```python
from build123d import *

# Parameters (mm, degrees)
CHAMFER1_SIZE                 = 1.5
TAP_DRILL_FOR_4_40_TAP1_D     = 2.2606
TAP_DRILL_FOR_4_40_TAP1_DEPTH = 8.89
TAP_DRILL_FOR_4_40_TAP1_TIP   = 0.679152758
TAP_DRILL_FOR_4_40_TAP2_D     = 2.2606
TAP_DRILL_FOR_4_40_TAP2_DEPTH = 8.89
TAP_DRILL_FOR_4_40_TAP2_TIP   = 0.679152758
SKETCH8_R                     = 1.524
CUT_EXTRUDE1_DEPTH            = 8.89
CIRPATTERN1_COUNT             = 6
SKETCH12_W                    = 20.7971
SKETCH12_H                    = 2
CUT_EXTRUDE3_DEPTH            = 2
FILLET1_R                     = 0.5


with BuildPart() as part:
    # Sketch3 → Revolve1 (revolve)
    with BuildSketch(Plane(origin=(0, 0, 0), x_dir=(1, 0, 0), z_dir=(0, 1, 0)), mode=Mode.PRIVATE) as revolve1_sk:
        Polygon((-10.39855, -111.125), (10.39855, -111.125), (10.39855, -107), (5.39855, -107), (5.39855, -100), (1.5875, -100), (1.5875, -101), (-1.5875, -101), (-1.5875, -100), (-5.39855, -100), (-5.39855, -107), (-10.39855, -107), align=None)
    revolve(revolve1_sk.sketch.rotate(Axis((0, 0, 0), (-1, 0, 0)), 180), axis=Axis((0, 0, 0), (-1, 0, 0)))

    # Chamfer1
    chamfer1_edges = [part.edges().sort_by_distance(p)[0] for p in [
        (5.39855, 0, 100),
    ]]
    chamfer(chamfer1_edges, length=CHAMFER1_SIZE)

    # Tap Drill for _4-40 Tap1
    with Locations(Plane(origin=(5.39855, -103.5, 0), x_dir=(0, 0, 1), z_dir=(1, 0, 0))):
        with Locations((0, 0), (89.633629292, -51.75), (-89.633629292, -51.75), (-89.633629292, -155.25), (0, -207), (89.633629292, -155.25)):
            Hole(TAP_DRILL_FOR_4_40_TAP1_D / 2, depth=TAP_DRILL_FOR_4_40_TAP1_DEPTH)
            with Locations((0, 0, -(TAP_DRILL_FOR_4_40_TAP1_DEPTH + TAP_DRILL_FOR_4_40_TAP1_TIP / 2))):  # 118° drill point
                Cone(0, TAP_DRILL_FOR_4_40_TAP1_D / 2, TAP_DRILL_FOR_4_40_TAP1_TIP, mode=Mode.SUBTRACT)

    # Tap Drill for _4-40 Tap2
    with Locations(Plane(origin=(-5.39855, -89.633629292, 51.75), x_dir=(0, 0, -1), z_dir=(-1, 0, 0))):
        with Locations((0, 0), (-51.75, -89.633629292), (0, -179.267258584), (103.5, -179.267258584), (155.25, -89.633629292), (103.5, 0)):
            Hole(TAP_DRILL_FOR_4_40_TAP2_D / 2, depth=TAP_DRILL_FOR_4_40_TAP2_DEPTH)
            with Locations((0, 0, -(TAP_DRILL_FOR_4_40_TAP2_DEPTH + TAP_DRILL_FOR_4_40_TAP2_TIP / 2))):  # 118° drill point
                Cone(0, TAP_DRILL_FOR_4_40_TAP2_D / 2, TAP_DRILL_FOR_4_40_TAP2_TIP, mode=Mode.SUBTRACT)

    # Sketch8 → Cut-Extrude1 (cut)
    with BuildSketch(Plane(origin=(0, 107.338507446, 28.761266387), x_dir=(-1, 0, 0), z_dir=(0, 0.9659258262890681, 0.25881904510252135))):
        with Locations(Location((-2.89855, 0, 0), (0, 0, 90))):
            Circle(SKETCH8_R)
        with Locations(Location((2.89855, 0, 0), (0, 0, 90))):
            Circle(SKETCH8_R)
    cut_extrude1 = extrude(amount=-CUT_EXTRUDE1_DEPTH, mode=Mode.SUBTRACT)

    # CirPattern1: Cut-Extrude1 ×6 about axis
    cirpattern1_axis = Axis((0, 0, 0), (1, 0, 0))
    for i in range(1, CIRPATTERN1_COUNT):
        add(cut_extrude1.rotate(cirpattern1_axis, i * 360 / CIRPATTERN1_COUNT), mode=Mode.SUBTRACT)

    # Sketch12 → Cut-Extrude3 (cut)
    with BuildSketch(Plane(origin=(10.39855, -9.685181913, -110.702135825), x_dir=(-1, 0, 0), z_dir=(0, -0.08715574274765833, -0.9961946980917457))):
        with Locations((10.39855, 1)):
            Rectangle(SKETCH12_W, SKETCH12_H)
        with Locations((10.39855, -1)):
            Rectangle(SKETCH12_W, SKETCH12_H)
    extrude(amount=-CUT_EXTRUDE3_DEPTH, mode=Mode.SUBTRACT)

    # Fillet1
    fillet1_edges = [part.edges().sort_by_distance(p)[0] for p in [
        (0, -11.676002575, -110.509893624),
        (0, -7.691223782, -110.858516595),
        (10.39855, -11.589631199, -109.522664284),
        (10.39855, -7.604852407, -109.871287255),
        (-10.39855, -7.604852407, -109.871287255),
        (-10.39855, -9.510870427, -108.709746429),
        (-10.39855, -11.589631199, -109.522664284),
        (0, -11.503259824, -108.535434944),
        (10.39855, -9.510870427, -108.709746429),
        (0, -7.518481031, -108.884057915),
    ]]
    fillet(fillet1_edges, radius=FILLET1_R)


solid = part.part
```
Model file for the job. Use its own axes, mm. A direction names the side the tool comes from. Coordinates: 2 decimals unless noted, no trailing zeros. Answer as a JSON object with one key per item and string values. Group by question number.
(1) Two-plate mould, pull along Y, no slides. Class faces 5 (the face through (10.399, -91, 58)), 6 (the face through (0.15, 4.84, 111.02)), 7 (the face through (2.73, -30.04, -95.38)), 8 (the face through (-7.93, 65.11, 84.91)): released by +Y, released by -Y, zero draft, split by the parting line, or undercut.
(2) Probe line 1 along Y through (x, z) = (3.4, 0) (3 decimals); line 2 along Y through (x, z) = (-1, -51.75); line 3 along Z through (x, y) = (2.5, 51.75). List the from-to ranges inside material, lowest first.
(3) Tool access for faces 1 (the face through (-10.399, -91, -58)), 2 (the face through (7.86, 65.11, 84.91)), 3 (the face through (-5.399, 71, 71)), 4 (the face through (-1.588, -23, 98)): list every direction of +Z, -Z, +X, -X, +Y, -Y with a clear straight run to the whole face (end or side of a thin tool).
(4) Flat gauge pins, fed straight in: pin 1 (3 mm diameter, centred on y = -51.75, z = 89.63, fed in from +X); pin 2 (5 mm diameter, centred on x = -1, y = -55, fed in from +Z); pin 3 (5 mm diameter, centred on x = 0, y = -20, fed in from +Z). Where does each tip first touch, or does it go through?
Geometry says:
{
 "1": {"face 5": "zero draft", "face 6": "split by the parting line", "face 7": "undercut", "face 8": "undercut"},
 "2": {"line 1": "y = -111.125 to -104.63, -102.37 to -100, 100 to 102.37, 104.63 to 111.125", "line 2": "y = -98.34 to -90.76, -88.5 to -86.73, 86.73 to 88.5, 90.76 to 98.34", "line 3": "z = -98.34 to -90.76, -88.5 to -85.57, 85.57 to 88.5, 90.76 to 98.34"},
 "3": {"face 1": "+Z, -Z, -X, +Y, -Y", "face 2": "+X", "face 3": "-X", "face 4": "none"},
 "4": {"pin 1": "stops at x = 5.4", "pin 2": "stops at z = 97.94", "pin 3": "stops at z = 109.74"}
}
